Read the model definition and answer for the solid it produces. Units are mm, in the model's axes. Give positions to 0.01 mm unless a question says otherwise; leave off trailing zeros. Order: outer loops, then holes, each group sorted by start corner. A loop starts at its lowest first (then second) coordinate and runs counter-clockwise, first axis right, second up. Notation, with made-up numbers: (-34.5, 21) - (20.5, 21) arc R26 cw to (20.5, 37) - close; hole circle Ø10 at (-10.75, -17.5). An arc over 180 degrees is marked (long way). Write each question's results on one line, items separated by ' | '. Start each with the question number.
Q1. For a pull along Z with two mould halves and no side action, classify faces 1 (the face through (-39, 5, 80)), 2 (the face through (0, 5, 39)), 3 (the face through (-37.83, 4.93, 49.76)), 4 (the face through (-41, 5, 0)) as +Z half, -Z half, draft (parallel to the pull), parting line (faces both ways), or undercut.
Q2. Find section A-A on z = 48. Give the vertices of the cut face in (x, y).
Q3. Find section B-B on x = -40. Give the vertices of the cut face in (y, z), and give its area (3 significant figures).
Q4. Find the intervals of material crossed by line 1 along Z through (x, y) = (-40, 6); line 2 along Z through (x, y) = (-47, 2.75); line 3 along X through (y, z) = (7.5, 31), in increasing order. Write a range as from..to.
Q5. Find section C-C on y = 3. Give the vertices of the cut face in (x, z).
Autodesk Inventor part; units mm, degrees
ref_plane "YZ Plane" through (0, 0, 0) normal (1, 0, 0) x (0, 1, 0)
ref_plane "XZ Plane" through (0, 0, 0) normal (0, 1, 0) x (-1, 0, 0)
ref_plane "XY Plane" through (0, 0, 0) normal (0, 0, 1) x (1, 0, 0)
sketch "Sketch1" plane through (0, 0, 0) normal (0, 1, 0) x (-1, 0, 0)
  line L0 (0, 0) -> (0, 80)
  line L1 (0, 80) -> (80, 80)
  line L2 (80, 80) -> (80, 0)
  line L3 (80, 0) -> (0, 0)
  circle A0 centre (40, 40) radius 10
  dimension "d0" = 80
extrude "Extrusion1" add sketch "Sketch1" along normal blind 10
properties part number "P1-5"
Working result:
1) face 1: +Z half | face 2: draft | face 3: undercut | face 4: -Z half
2) outline: (-80, 0) - (-46, 0) - (-46, 10) - (-80, 10) - close; (-34, 0) - (0, 0) - (0, 10) - (-34, 10) - close
3) outline: (0, 0) - (10, 0) - (10, 30) - (0, 30) - close; (0, 50) - (10, 50) - (10, 80) - (0, 80) - close | area: 600 mm²
4) line 1: 0..30, 50..80 | line 2: 0..32.86, 47.14..80 | line 3: -80..-44.36, -35.64..0
5) outline: (-80, 0) - (0, 0) - (0, 80) - (-80, 80) - close; hole circle Ø20 at (-40, 40)
